from build123d import *

# Parameters (mm, degrees)
F2_R = 13.0661787558
F3_R = 30.5326661472
F4_R = 6.4496868792
F5_T = 1.27


# Not quite as in the source:
# - a shell that OpenCascade refuses in one call is made with other operations: the cavity is built on its own and cut out


with BuildPart() as f1:
    # F0 (on Front) → F1 (revolve)
    with BuildSketch(Plane.XZ):
        Polygon((0, 58.8393360376), (0, 0), (12.5450463966, 0), (19.0413612872, 16.967702657), (6.6549694166, 36.8729744223), (7.8558586538, 56.0485236347), (12.1103581041, 58.8393360376), align=None)
    revolve(axis=Axis((0, 0, 29.4196680188), (0, 0, -1)))

    # F2
    f2_edges = [f1.edges().sort_by_distance(p)[0] for p in [
        (-19.041361, 0, 16.967703),
    ]]
    fillet(f2_edges, radius=F2_R)

    # F3
    f3_edges = [f1.edges().sort_by_distance(p)[0] for p in [
        (-6.654969, 0, 36.872974),
    ]]
    fillet(f3_edges, radius=F3_R)

    # F4
    f4_edges = [f1.edges().sort_by_distance(p)[0] for p in [
        (-7.855859, 0, 56.048524),
    ]]
    fillet(f4_edges, radius=F4_R)

    # F5: shell of thickness 1.27, made by hand


with BuildPart() as f5_core1:
    # F5_t2: copy of F1
    add(f1.part)

    # the walls: a layer under each face that stays
    f5_faces = [f5_core1.faces().sort_by_distance(p)[0] for p in [
        (-7.4598050795, 0, 49.724422652),
        (-8.5147014286, 0, 55.6656825004),
        (-8.1326981188, 0, 37.2456508864),
        (-11.3320158511, 0, 58.3287689924),
        (-13.7131490398, 0, 25.5302860078),
        (-17.5243000505, 0, 16.8223934121),
        (-14.6325546639, 0, 5.4523557079),
        (0, 0, 0),
    ]]
    thicken(f5_faces, amount=-F5_T, mode=Mode.SUBTRACT)


with BuildPart() as f1_1:
    add(f1.part)

    # what is left inside the walls is the cavity
    f5_cavity = [f5_core1.part.solids().sort_by_distance(p)[0] for p in [
        (-8.12206, -14.071681, 16.700091),
    ]]
    add(f5_cavity, mode=Mode.SUBTRACT)


solid = f1_1.part
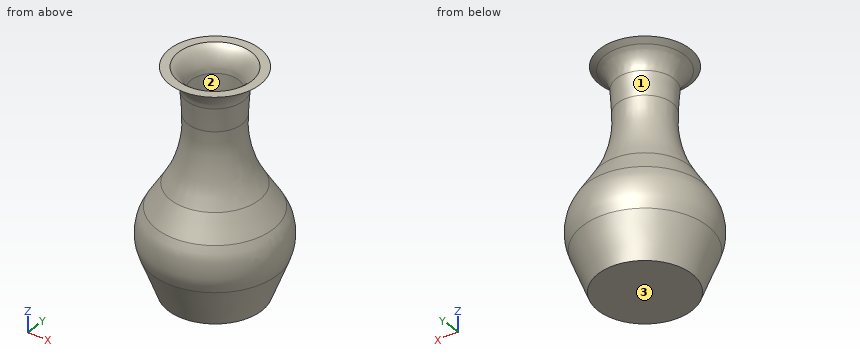
Geometry: final body of the model. Coordinates: model frame, mm. Face numbers are marked on the shaded views. Round coordinates to 2 decimals unless told otherwise and drop trailing zeros. Put each result on its own line as item: value. Start each with the question number.
Q1. Line query: probe 1 along Z at (x, y) = (-11, 3.5); probe 2 along Z at (x, y) = (-1.5, 4.5); probe 3 along X at (y, z) = (4, 55.5). Output: solid intervals per line, ascending.
Q2. Pull-direction query (Z, two-part tool) for the marked faces 1, 2 and 3; classes: +Z half, -Z half, draft (parallel to the pull), parting line (faces both ways), or undercut.
Q3. Section A-A on x = 9. Give the number of separate pieces and of enclosed holes in the cut face, and give its area (3 significant figures).
Q4. First-contact query: pin 1 (4 mm diameter, centred on x = -9.5, y = 11.5, fed in from +Z); pin 2 (10 mm diameter, centred on y = 13.5, z = 19, fed in from +X); pin 3 (11.5 mm diameter, centred on x = -0.5, y = 5, fed in from +Z); pin 4 (12 mm diameter, centred on x = -8, z = 48, fed in from -Y). Flat tips, straight axial feed; report the tip coordinate or a pass-through.
Ans:
1. probe 1: z = 0 to 1.27, 26.61 to 29.03, 58.47 to 58.84
1. probe 2: z = 0 to 1.27
1. probe 3: x = -7.41 to -5.76, 5.76 to 7.41
2. face 1: undercut
2. face 2: +Z half
2. face 3: -Z half
3. separate pieces: 2
3. enclosed holes: 1
3. area: 179 mm2
4. pin 1: stops at z = 26.81
4. pin 2: stops at x = 15.1
4. pin 3: stops at z = 58.84
4. pin 4: stops at y = -7.12
